Geometry: final body of the model. Coordinates: model frame, mm. Face numbers are marked on the shaded views. A direction names the side the tool comes from. Give positions to 0.01 mm unless a question says otherwise; leave off trailing zeros. Write each loop counter-clockwise with the first axis right and the second up, starting at its lowest first coordinate (ties: lowest second). Pieces come first, ordered by that corner, then holes. Notation, with made-up numbers: M -34.5,-2 L -4.5,-2 A33 ccw -4.5,35 Z; hole C 50,-36 d6. An arc over 180 degrees is marked long. Use a Markdown table: item, result. Add a question column.
(1) Pin query (flat end, axial travel): pin 1 Ø5 at (x, z) = (42.5, 9) entering from +Y; pin 2 Ø1.5 at (x, z) = (19, 12.5) entering from -Y; pin 3 Ø4 at (x, z) = (49.5, 6) entering from +Y. Return the tip coordinate at first contact, or that it passes through.
(2) Reachability of the marked faces 4 and 5 from +Z, -Z, +X, -X, +Y, -Y: full face, straight path, thin tool, end or side. Return the list, or none.
(3) Draft query along X for the marked faces 1, 2 and 3. Return one class per face: released by +X, released by -X, zero draft, split by the parting line, or undercut.
(4) Material intervals for L1, parallel to X at y = 16.9, z = 0.9; L2, parallel to Y at x = 2.9, z = 0.95; L3, parallel to Y at x = 39.5, z = 7.75, sorted ascending.
(5) Cut plane B-B (x = 9). Output: boundary loops of the cut face in (y, z).
(6) Cut plane A-A (x = 2.9). Output: boundary loops of the cut face in (y, z).
```python
from build123d import *

# Parameters (mm, degrees)
BOSS_EXTRUDE1_DEPTH = 17.6
SKETCH4_W           = 4.750417
SKETCH4_H           = 13.7
CUT_EXTRUDE1_DEPTH  = 5.8
SKETCH5_R           = 1.6
CUT_EXTRUDE2_DEPTH  = 17.8
BOSS_EXTRUDE2_DEPTH = 107
FILLET1_R           = 4
CHAMFER1_SIZE       = 0.5


with BuildPart() as part:
    # Sketch3 → Boss-Extrude1 (new body)
    with BuildSketch(Plane.XY):
        with BuildLine():
            Line((0, 0), (0, 19.8))
            Line((0, 19.8), (4.750417, 19.8))
            Line((4.750417, 19.8), (4.750417, 6))
            Line((4.750417, 6), (21.75, 6))
            ThreePointArc((21.75, 6), (22.769877953, 2.926324181), (25.730987279, 1.615040214))
            Line((25.730987279, 1.615040214), (25.730987279, 0))
            Line((25.730987279, 0), (0, 0))
        make_face()
    extrude(amount=BOSS_EXTRUDE1_DEPTH)

    # Sketch4 → Cut-Extrude1 (cut)
    with BuildSketch(Plane(origin=(0, 19.8, 0), x_dir=(1, 0, 0), z_dir=(0, 1, 0))):
        with Locations((2.3752085, -8.8)):
            Rectangle(SKETCH4_W, SKETCH4_H)
    extrude(amount=-CUT_EXTRUDE1_DEPTH, mode=Mode.SUBTRACT)

    # Sketch5 → Cut-Extrude2 (cut)
    with BuildSketch(Plane(origin=(0, 0, 0), x_dir=(-1, 0, 0), z_dir=(0, 0, -1))):
        with Locations(Location((-2.9, 16.9, 0), (0, 0, 180))):
            Circle(SKETCH5_R)
    extrude(amount=-CUT_EXTRUDE2_DEPTH, mode=Mode.SUBTRACT)

    # Sketch6 → Boss-Extrude2 (add)
    with BuildSketch(Plane.XZ):
        with BuildLine():
            Line((25.730987279, 11.799763823), (25.730987279, 5.800480479))
            ThreePointArc((25.730987279, 5.800480479), (22.684620888, 8.800122151), (25.730987279, 11.799763823))
        make_face()
    extrude(amount=BOSS_EXTRUDE2_DEPTH)

    # Fillet1
    fillet1_edges = [part.edges().sort_by_distance(p)[0] for p in [
        (22.684620888, 0, 8.800122151),
    ]]
    fillet(fillet1_edges, radius=FILLET1_R)

    # Chamfer1
    # the kernel refuses this chamfer: 0.5 mm, written as the material it takes off along each edge
    with BuildSketch(Plane(origin=(2.9, 16.9, 17.6), x_dir=(1, 0, 0), z_dir=(0, 1, 0))) as chamfer1_piece_1:
        Polygon((1.6 + CHAMFER1_SIZE, 0), (1.6, CHAMFER1_SIZE), (1.6, 0), align=None)
    revolve(axis=Axis((2.9, 16.9, 17.6), (0, 0, -1)), mode=Mode.SUBTRACT)

    # Mirror4: part across plane


with BuildPart() as part_1:
    add(part.part)
    add(part.part.mirror(Plane(origin=(25.730987279, 0, 17.6), x_dir=(0, 0, 1), z_dir=(-1, 0, 0))))


solid = part_1.part
```
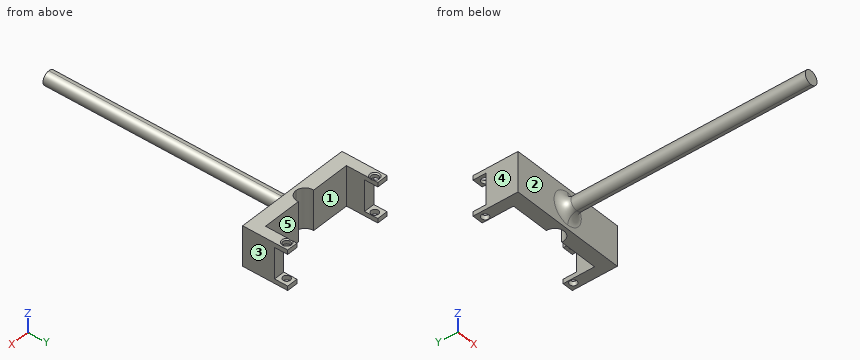
Answer list:
| question | item | result |
|---|---|---|
| 1 | pin 1 | y = 6 |
| 1 | pin 2 | y = 0 |
| 1 | pin 3 | y = 14 |
| 2 | face 4 | +Z, -Z, -X, +Y, -Y |
| 2 | face 5 | +Z, -Z, +Y |
| 3 | face 1 | undercut |
| 3 | face 2 | zero draft |
| 3 | face 3 | released by +X |
| 4 | L1 | 0 to 1.3, 4.5 to 4.75, 46.71 to 46.96, 50.16 to 51.46 |
| 4 | L2 | 0 to 15.3, 18.5 to 19.8 |
| 4 | L3 | 0 to 6 |
| 5 | outline | M 0,0 L 6,0 L 6,17.6 L 0,17.6 Z |
| 6 | outline | M 0,0 L 15.3,0 L 15.3,1.95 L 14,1.95 L 14,15.65 L 15.3,15.65 L 15.3,17.1 L 14.8,17.6 L 0,17.6 Z; M 18.5,0 L 19.8,0 L 19.8,1.95 L 18.5,1.95 Z; M 18.5,15.65 L 19.8,15.65 L 19.8,17.6 L 19,17.6 L 18.5,17.1 Z |
